```python
from build123d import *

# Parameters (mm, degrees)
SKETCH058_R        = 45
SKETCH058_R_2      = 35
SKETCH058_R_3      = 1.125
PAD018_DEPTH       = 3
SKETCH059_R        = 2
POCKET040_DEPTH    = 2
CHAMFER010_1_SIZE2 = 0.75
CHAMFER010_1_SIZE  = 1.5
CHAMFER010_2_SIZE2 = 0.75
CHAMFER010_2_SIZE  = 1.5
CHAMFER010_3_SIZE2 = 0.75
CHAMFER010_3_SIZE  = 1.5
CHAMFER010_4_SIZE2 = 0.75
CHAMFER010_4_SIZE  = 1.5
CHAMFER011_SIZE    = 0.49


with BuildPart() as part:
    # Sketch058 (on Face1 of ShapeBinder010) → Pad018 (new body)
    with BuildSketch(Plane(origin=(248, 250.5, 0), x_dir=(1, 0, 0), z_dir=(0, -1, 0))):
        with Locations((-124, 113.916594)):
            Circle(SKETCH058_R)
        with Locations((-124, 113.916594)):
            Circle(SKETCH058_R_2, mode=Mode.SUBTRACT)
        with Locations((-162.75, 113.916594)):
            Circle(SKETCH058_R_3, mode=Mode.SUBTRACT)
        with Locations((-124, 152.666594)):
            Circle(SKETCH058_R_3, mode=Mode.SUBTRACT)
        with Locations((-85.25, 113.916594)):
            Circle(SKETCH058_R_3, mode=Mode.SUBTRACT)
        with Locations((-124, 75.166594)):
            Circle(SKETCH058_R_3, mode=Mode.SUBTRACT)
    extrude(amount=PAD018_DEPTH)

    # Sketch059 (on Face8 of Pad018) → Pocket040 (cut)
    with BuildSketch(Plane(origin=(248, 247.5, 0), x_dir=(1, 0, 0), z_dir=(0, -1, 0))):
        with Locations((-85.25, 113.916594)):
            Circle(SKETCH059_R)
        with Locations((-124, 152.666594)):
            Circle(SKETCH059_R)
        with Locations((-162.75, 113.916594)):
            Circle(SKETCH059_R)
        with Locations((-124, 75.166594)):
            Circle(SKETCH059_R)
    extrude(amount=-POCKET040_DEPTH, mode=Mode.SUBTRACT)

    # Chamfer010 1
    chamfer010_1_edges = [part.edges().sort_by_distance(p)[0] for p in [
        (160.75, 249.5, 113.916594),
    ]]
    chamfer010_1_side = part.faces().sort_by_distance((160.75, 248.5, 113.916594))[0]
    chamfer(chamfer010_1_edges, length=CHAMFER010_1_SIZE, length2=CHAMFER010_1_SIZE2, reference=chamfer010_1_side)

    # Chamfer010 2
    chamfer010_2_edges = [part.edges().sort_by_distance(p)[0] for p in [
        (83.25, 249.5, 113.916594),
    ]]
    chamfer010_2_side = part.faces().sort_by_distance((83.25, 248.5, 113.916594))[0]
    chamfer(chamfer010_2_edges, length=CHAMFER010_2_SIZE, length2=CHAMFER010_2_SIZE2, reference=chamfer010_2_side)

    # Chamfer010 3
    chamfer010_3_edges = [part.edges().sort_by_distance(p)[0] for p in [
        (122, 249.5, 152.666594),
    ]]
    chamfer010_3_side = part.faces().sort_by_distance((122, 248.5, 152.666594))[0]
    chamfer(chamfer010_3_edges, length=CHAMFER010_3_SIZE, length2=CHAMFER010_3_SIZE2, reference=chamfer010_3_side)

    # Chamfer010 4
    chamfer010_4_edges = [part.edges().sort_by_distance(p)[0] for p in [
        (122, 249.5, 75.166594),
    ]]
    chamfer010_4_side = part.faces().sort_by_distance((122, 248.5, 75.166594))[0]
    chamfer(chamfer010_4_edges, length=CHAMFER010_4_SIZE, length2=CHAMFER010_4_SIZE2, reference=chamfer010_4_side)

    # Chamfer011
    chamfer011_edges = [part.edges().sort_by_distance(p)[0] for p in [
        (79, 250.5, 113.916594),
        (79, 247.5, 113.916594),
        (122, 247.5, 152.666594),
        (83.25, 247.5, 113.916594),
        (122, 247.5, 75.166594),
        (89, 247.5, 113.916594),
        (160.75, 247.5, 113.916594),
    ]]
    chamfer(chamfer011_edges, length=CHAMFER011_SIZE)


solid = part.part
```
Part model, mm, in its own coordinate system. Coordinates: 2 decimals unless noted, no trailing zeros. Order: outer loops, then holes, each group sorted by start corner. A loop starts at its lowest first (then second) coordinate and runs counter-clockwise, first axis right, second up. Notation, with made-up numbers: (14.25, -4.5) - (21.25, -4.5) arc R30 cw to (21.25, 27.5) - close; hole circle Ø11 at (15, 33). An arc over 180 degrees is marked (long way). Return JSON: item names as keys, results as strings. Group by question number.
Item 1: Drill centre lines: probe 1 along Z at (x, y) = (124, 249.75); probe 2 along X at (y, z) = (247.75, 112); probe 3 along X at (y, z) = (250.15, 90). Where is each one in solid material? Low to high. Write a range as from..to.
Item 2: Pull direction X, two halves, no side cores. Call faces 1 (the face through (110.6, 247.5, 147.1)), 2 (the face through (88.29, 249.014, 86.535)), 3 (the face through (161.86, 250.01, 113.23)): pulls with the +X half, pulls with the -X half, needs draft (parallel to the pull), parting line crosses it, or undercut.
Item 3: Cut at A-A (x = 124). State how many separate pieces and enclosed holes the cut face has, plus the area to 3 significant figures.
Item 4: Pin check, flat tips, straight feed: pin 1 (2.5 mm diameter, centred on x = 162.75, z = 113.92, fed in from +Y); pin 2 (2 mm diameter, centred on x = 123.5, z = 75.5, fed in from -Y); pin 3 (3 mm diameter, centred on x = 124, z = 152.67, fed in from -Y); pin 4 (1.8 mm diameter, centred on x = 85.25, z = 113.92, fed in from -Y). Stop position of each tip, or through.
Item 5: Cut at B-B (y = 249). List the corners of the cut face in (x, z).
Check values:
{
 "1": {"probe 1": "z = 68.92..74.04, 76.29..78.92, 148.92..151.54, 153.79..158.92", "probe 2": "x = 79.28..84.09, 86.41..88.81, 159.19..161.59, 163.91..168.72", "probe 3": "x = 86.05..98.45, 149.55..161.95"},
 "2": {"face 1": "needs draft", "face 2": "parting line crosses it", "face 3": "undercut"},
 "3": {"separate pieces": "4", "enclosed holes": "0", "area": "40.5 mm2"},
 "4": {"pin 1": "stops at y = 250.5", "pin 2": "stops at y = 248.8", "pin 3": "stops at y = 248.99", "pin 4": "passes through"},
 "5": {"outline": "circle Ø90 at (124, 113.92); hole circle Ø3 at (85.25, 113.92); hole circle Ø70 at (124, 113.92); hole circle Ø3 at (124, 75.17); hole circle Ø3 at (124, 152.67); hole circle Ø3 at (162.75, 113.92)"}
}
